CAD build for the part. Positions are in the model's coordinates, mm. A direction names the side the tool comes from. Coordinates: 2 decimals unless noted, no trailing zeros. Loops run counter-clockwise (first coordinate to the right, second up) from the corner with the lowest first, then second, coordinate; pieces in that order, holes last. Notation, with made-up numbers: (36, 28) - (53, 28) arc R8 cw to (53, 37) - close; hole circle Ø4 at (44.25, 71). An arc over 180 degrees is marked (long way). Put each result on its own line as item: value.
```python
from build123d import *

# Parameters (mm, degrees)
SKETCH1_R           = 23
BOSS_EXTRUDE1_DEPTH = 40
SKETCH2_R           = 21.05
BOSS_EXTRUDE2_DEPTH = 22.3
BOSS_EXTRUDE3_START = 4.2
SKETCH3_R           = 21.05
BOSS_EXTRUDE3_DEPTH = 4.2
FILLET1_R           = 2
SKETCH4_R           = 7.5
BOSS_EXTRUDE4_DEPTH = 4.4
FILLET2_R           = 2
SKETCH5_R           = 2.5
BOSS_EXTRUDE5_DEPTH = 17
FILLET3_R           = 0.5
BOSS_EXTRUDE6_START = 4
SKETCH6_R           = 7.5
BOSS_EXTRUDE6_DEPTH = 4
SKETCH7_R           = 2.25
CUT_EXTRUDE1_DEPTH  = 0.7


with BuildPart() as part:
    # Sketch1 → Boss-Extrude1 (new body)
    with BuildSketch(Plane.XY):
        Circle(SKETCH1_R)
    extrude(amount=BOSS_EXTRUDE1_DEPTH)

    # Sketch2 → Boss-Extrude2 (add)
    with BuildSketch(Plane.XY.offset(40)):
        Circle(SKETCH2_R)
    extrude(amount=BOSS_EXTRUDE2_DEPTH)

    # Sketch3 → Boss-Extrude3 (add)
    with BuildSketch(Plane(origin=(0, 0, 0), x_dir=(-1, 0, 0), z_dir=(0, 0, -1)).offset(BOSS_EXTRUDE3_START)):
        with Locations(Location((0, 0, 0), (0, 0, 180))):
            Circle(SKETCH3_R)
    extrude(amount=-BOSS_EXTRUDE3_DEPTH)

    # Fillet1
    fillet1_edges = [part.edges().sort_by_distance(p)[0] for p in [
        (-21.05, 0, -4.2),
    ]]
    fillet(fillet1_edges, radius=FILLET1_R)

    # Sketch4 → Boss-Extrude4 (add)
    with BuildSketch(Plane(origin=(0, 0, -4.2), x_dir=(-1, 0, 0), z_dir=(0, 0, -1))):
        Circle(SKETCH4_R)
    extrude(amount=BOSS_EXTRUDE4_DEPTH)

    # Fillet2
    fillet2_edges = [part.edges().sort_by_distance(p)[0] for p in [
        (7.5, 0, -8.6),
    ]]
    fillet(fillet2_edges, radius=FILLET2_R)

    # Sketch5 → Boss-Extrude5 (add)
    with BuildSketch(Plane(origin=(0, 0, -8.6), x_dir=(-1, 0, 0), z_dir=(0, 0, -1))):
        Circle(SKETCH5_R)
    extrude(amount=BOSS_EXTRUDE5_DEPTH)

    # Fillet3
    fillet3_edges = [part.edges().sort_by_distance(p)[0] for p in [
        (2.5, 0, -25.6),
    ]]
    fillet(fillet3_edges, radius=FILLET3_R)

    # Sketch6 → Boss-Extrude6 (add)
    with BuildSketch(Plane.XY.offset(62.3).offset(BOSS_EXTRUDE6_START)):
        with Locations(Location((0, 0, 0), (0, 0, 180))):
            Circle(SKETCH6_R)
    extrude(amount=-BOSS_EXTRUDE6_DEPTH)

    # Sketch7 → Cut-Extrude1 (cut)
    with BuildSketch(Plane(origin=(0, 0, -4.2), x_dir=(-1, 0, 0), z_dir=(0, 0, -1))):
        with Locations((0, 14.5)):
            Circle(SKETCH7_R)
        with Locations((14.5, 0)):
            Circle(SKETCH7_R)
        with Locations((0, -14.5)):
            Circle(SKETCH7_R)
        with Locations((-14.5, 0)):
            Circle(SKETCH7_R)
    extrude(amount=-CUT_EXTRUDE1_DEPTH, mode=Mode.SUBTRACT)


solid = part.part
```
Q1. Slice it at A-A, the plane z = 44. Give the cut face in (x, y).
Determined:
outline: circle Ø42.1 at (0, 0)
Q2. Tool access for faces 1 (the flat face through (0, 0, 66.3)), 2 (the flat face through (0, -14, -3.5)), 3 (the cylindrical face through (20.08, 6.32, 50.99)): list every direction of +Z, -Z, +X, -X, +Y, -Y with a clear straight run to the whole face (end or side of a thin tool).
Determined:
face 1: +Z, +X, -X, +Y, -Y
face 2: -Z
face 3: +Z
Q3. Pin check, flat tips, straight feed: pin 1 Ø2 at (x, y) = (-14.5, -0.5) entering from -Z; pin 2 Ø4 at (x, z) = (-17, 21.5) entering from -Y; pin 3 Ø1.5 at (y, z) = (-15.5, 7.5) entering from -X. Stop position of each tip, or through.
Determined:
pin 1: z = -3.5
pin 2: y = -17.44
pin 3: x = -17.65
Q4. Mould opens along Y. For faces 4 (the flat face through (8, 0, -4.2)), 5 (the flat face through (0, 15, -3.5)), 6 (the cylindrical face through (12.354, 0.676, -3.855)), 7 (the cylindrical face through (-2.994, 22.804, 19.72)) say: +Y half, -Y half, draft (parallel to the pull), parting line (faces both ways), or undercut.
Determined:
face 4: draft
face 5: undercut
face 6: undercut
face 7: parting line
Q5. Slice it at B-B, the plane z = 14.5. Give the cut face in (x, y), then the cut area to 3 significant figures.
Determined:
outline: circle Ø46 at (0, 0)
area: 1,660 mm2
Q6. Wall check: L1, parallel to Y at x = 0, z = -3.95; L2, parallel to Y at x = 0, z = -3.9; L3, parallel to Y at x = 14.5, z = -3.8. Give the ranges that are in metal, low to high. Write a range as from..to.
Determined:
L1: -20.02..-16.75, -12.25..12.25, 16.75..20.02
L2: -20.1..-16.75, -12.25..12.25, 16.75..20.1
L3: -14.14..-2.25, 2.25..14.14
